Check sheet for the modelled part. Datum: model origin and axes. Units: mm. A direction names the side the tool comes from. Round coordinates to 2 decimals unless told otherwise and drop trailing zeros. Order: outer loops, then holes, each group sorted by start corner. A loop starts at its lowest first (then second) coordinate and runs counter-clockwise, first axis right, second up.
(1) Tool access check on faces 1 (the flat face through (2, -3, -2)), 2 (the flat face through (0, -6, -5.883)). Record the directions out of +Z, -Z, +X, -X, +Y, -Y that give a thin tool (end or side, any length) a straight path to the whole face; none if there is none.
(2) Thickness scan on probe 1 along Z at (x, y) = (0, -9.25); probe 2 along Z at (x, y) = (0, -0.95); probe 3 along Y at (x, z) = (-2.25, -1.5). Record the ranges inside material, lowest first.
(3) Sectioned sample at A-A, the plane z = 0. Enter the section's corners in (x, y).
(4) Sectioned sample at D-D, the plane z = 4.25. Enter the section's corners in (x, y).
(5) Sectioned sample at C-C, the plane y = -3.75. Enter the section's corners in (x, z).
(6) Sectioned sample at B-B, the plane x = 0. Enter the section's corners in (y, z).
(7) Mould release check, pull along X, two halves, no side actions. Record for faces 3 (the flat face through (-4, -11, 4.53)), 4 (the flat face through (3, -11.5, -3)), 5 (the flat face through (5.794, -6, 0)): released by +X, released by -X, zero draft, split by the parting line, or undercut.
```python
from build123d import *

# Parameters (mm, degrees)
F0_W      = 15.221721
F0_H      = 54.359732
F1_DEPTH  = 11.5
F3_D      = 7.5
F4_W      = 42.202285
F4_H      = 45.044836
F5_DEPTH  = 25
F6_W      = 6.489188
F6_H      = 15.716003
F7_DEPTH  = 14
F8_R      = 4.527333
F8_R_2    = 2.346749
F9_DEPTH  = 3
F10_W     = 1.5
F10_H     = 1.5
F11_DEPTH = 2


with BuildPart() as f1:
    # F0 (on Front) → F1 (new body)
    with BuildSketch(Plane.XZ):
        with Locations((-1.816982, -22.036255)):
            Rectangle(F0_W, F0_H)
    extrude(amount=F1_DEPTH)

    # F3 (through all)
    with Locations(Plane(origin=(0, 0, 0), x_dir=(1, 0, 0), z_dir=(0, 1, 0))):
        with Locations((0, 0)):
            Hole(F3_D / 2)

    # F4 (on Front) → F5 (cut)
    with BuildSketch(Plane.XZ):
        with Locations((0.021285, -28.405259)):
            Rectangle(F4_W, F4_H)
    extrude(amount=F5_DEPTH, mode=Mode.SUBTRACT)

    # F6 (on face) → F7 (cut)
    with BuildSketch(Plane.XZ.offset(11.5)):
        with Locations((-8.758753, -0.702533)):
            Rectangle(F6_W, F6_H)
    extrude(amount=-F7_DEPTH, mode=Mode.SUBTRACT)

    # F8 (on face) → F9 (join)
    with BuildSketch(Plane(origin=(0, 0, 0), x_dir=(-1, 0, 0), z_dir=(0, 1, 0))):
        Circle(F8_R)
        Circle(F8_R_2, mode=Mode.SUBTRACT)
    extrude(amount=-F9_DEPTH)

    # F10 (on face) → F11 (cut)
    with BuildSketch(Plane.XZ.offset(11.5)):
        with Locations((-4.104478, 3.780475)):
            Rectangle(F10_W, F10_H)
        with Locations((4.16695, -4.533809)):
            Rectangle(F10_W, F10_H)
    extrude(amount=-F11_DEPTH, mode=Mode.SUBTRACT)


solid = f1.part
```
Derived:
1. face 1: -Y
1. face 2: -Z, +X, -X, +Y, -Y
2. probe 1: z = -5.88 to -3.75, 3.75 to 5.14
2. probe 2: z = -5.88 to -2.35, 2.35 to 5.14
2. probe 3: y = -3 to 0
3. outline: (-5.51, -11.5) - (-3.75, -11.5) - (-3.75, -3) - (-2.35, -3) - (-2.35, 0) - (-5.51, 0) - close; (2.35, -3) - (3.75, -3) - (3.75, -11.5) - (5.79, -11.5) - (5.79, 0) - (2.35, 0) - close
4. outline: (-5.51, -11.5) - (-4.85, -11.5) - (-4.85, -9.5) - (-3.35, -9.5) - (-3.35, -11.5) - (5.79, -11.5) - (5.79, 0) - (-5.51, 0) - close
5. outline: (-5.51, -5.88) - (5.79, -5.88) - (5.79, 5.14) - (-5.51, 5.14) - close; hole circle Ø7.5 at (0, 0)
6. outline: (-11.5, -5.88) - (0, -5.88) - (0, -2.35) - (-3, -2.35) - (-3, -3.75) - (-11.5, -3.75) - close; (-11.5, 3.75) - (-3, 3.75) - (-3, 2.35) - (0, 2.35) - (0, 5.14) - (-11.5, 5.14) - close
7. face 3: undercut
7. face 4: zero draft
7. face 5: released by +X
